Source: three-view drawing plus pictorial views. Frame: mm from the lowest corner of the part. A direction names the side the tool comes from. Give positions to 0.01 mm unless a question says otherwise; leave off trailing zeros. Loops run counter-clockwise (first coordinate to the right, second up) from the corner with the lowest first, then second, coordinate; pieces in that order, holes last.
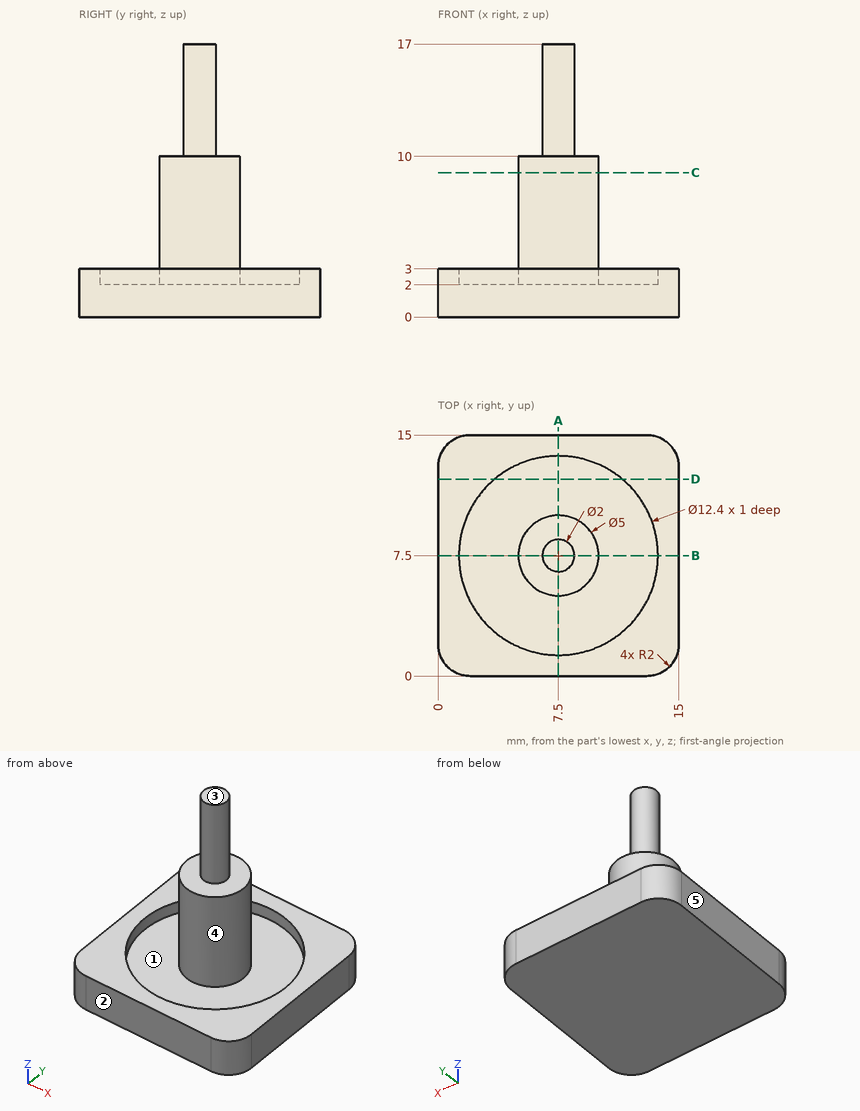
(1) Ray query, probe 1 along Y at (x, z) = (7.5, 2.35); probe 2 along Z at (x, y) = (11, 13.5); probe 3 along Z at (x, y) = (5, 12.5). Return the intervals inside material, ascending.
Values follow:
probe 1: y = 0 to 1.3, 5 to 10, 13.7 to 15
probe 2: z = 0 to 3
probe 3: z = 0 to 2
(2) Cut plane C-C (z = 9). Return the cut outline in (x, y), and give its area (3 significant figures).
Values follow:
outline: circle Ø5 at (7.5, 7.5)
area: 19.6 mm2
(3) Mould query, pull axis Y, two halves, no side actions, for the marked faces 1, 2 and 3. Classes: +Y half, -Y half, draft (parallel to the pull), parting line (faces both ways), or undercut.
Values follow:
face 1: undercut
face 2: -Y half
face 3: draft
(4) Reachability of the marked faces 4 and 5 from +Z, -Z, +X, -X, +Y, -Y: full face, straight path, thin tool, end or side. Return the list, or none.
Values follow:
face 4: +Z
face 5: +Z, -Z, -X, +Y, -Y
(5) Cut plane A-A (x = 7.5). Return the cut outline in (y, z).
Values follow:
outline: (0, 0) - (15, 0) - (15, 3) - (13.7, 3) - (13.7, 2) - (10, 2) - (10, 10) - (8.5, 10) - (8.5, 17) - (6.5, 17) - (6.5, 10) - (5, 10) - (5, 2) - (1.3, 2) - (1.3, 3) - (0, 3) - close
(6) Cut plane D-D (y = 12.25). Return the cut outline in (x, z).
Values follow:
outline: (0, 0) - (15, 0) - (15, 3) - (11.48, 3) - (11.48, 2) - (3.52, 2) - (3.52, 3) - (0, 3) - close
(7) Pin query (flat end, axial travel): pin 1 Ø5 at (y, z) = (7.5, 2) entering from -X; pin 2 Ø4 at (x, y) = (12, 6) entering from +Z. Return the tip coordinate at first contact, or that it passes through.
Values follow:
pin 1: stops at x = 0
pin 2: stops at z = 3
